Geometry: final body of the model. Coordinates: model frame, mm. Give positions to 0.01 mm unless a question says otherwise; leave off trailing zeros. Order: outer loops, then holes, each group sorted by start corner. A loop starts at its lowest first (then second) coordinate and runs counter-clockwise, first axis right, second up. Notation, with made-up numbers: (22.25, -8.5) - (66.25, -8.5) arc R33 cw to (66.25, 26.5) - close; hole circle Ø4 at (50.5, 66). An arc over 180 degrees is marked (long way). Use one line per item in the form item = value.
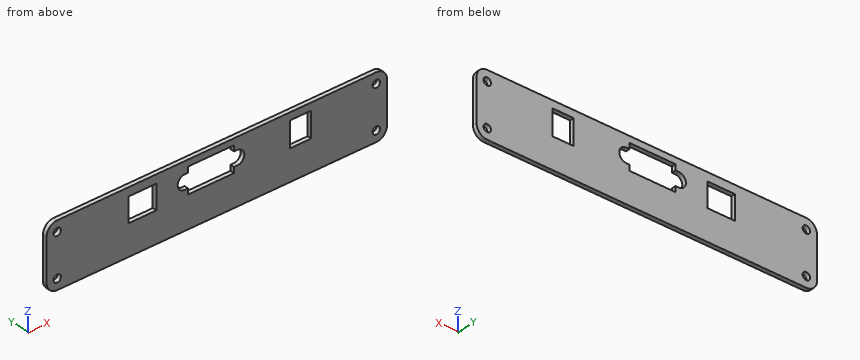
from build123d import *

# Parameters (mm, degrees)
SKETCH017_W          = 160
SKETCH017_H          = 30
PAD014_DEPTH         = 2
FILLET_R             = 5
SKETCH018_R          = 1.75
SKETCH018_W          = 13
SKETCH018_H          = 11.5
SKETCH018_W_2        = 10
SKETCH018_H_2        = 12
POCKET009_DEPTH      = 2.001
POCKET009_DEPTH_BACK = 0.001


with BuildPart() as part:
    # Sketch017 → Pad014 (new body)
    with BuildSketch(Plane.XZ):
        with Locations((0, 0.5)):
            Rectangle(SKETCH017_W, SKETCH017_H)
    extrude(amount=PAD014_DEPTH)

    # Fillet
    fillet_edges = [part.edges().sort_by_distance(p)[0] for p in [
        (80, -1, 15.5),
        (80, -1, -14.5),
        (-80, -1, 15.5),
        (-80, -1, -14.5),
    ]]
    fillet(fillet_edges, radius=FILLET_R)

    # Sketch018 (on Face5 of Pad014) → Pocket009 (cut, two sides)
    with BuildSketch(Plane(origin=(0, 0, 0), x_dir=(1, 0, 0), z_dir=(0, 1, 0))) as pocket009_sk:
        with Locations((-75, 9.5)):
            Circle(SKETCH018_R)
        with Locations((-75, -10.5)):
            Circle(SKETCH018_R)
        with Locations((75, 9.5)):
            Circle(SKETCH018_R)
        with Locations((75, -10.5)):
            Circle(SKETCH018_R)
        with BuildLine():
            Line((8.085, -12.5), (-13.515, -12.5))
            Line((-13.515, -12.5), (-13.515, -9.85))
            Line((-13.515, -9.85), (-15.015, -9.85))
            ThreePointArc((-15.015, -3.15), (-18.365, -6.5), (-15.015, -9.85))
            Line((-13.515, -3.15), (-15.015, -3.15))
            Line((-13.515, -0.5), (-13.515, -3.15))
            Line((8.085, -0.5), (-13.515, -0.5))
            Line((8.085, -3.15), (8.085, -0.5))
            Line((9.585, -3.15), (8.085, -3.15))
            ThreePointArc((9.585, -9.85), (12.935, -6.5), (9.585, -3.15))
            Line((8.085, -9.85), (9.585, -9.85))
            Line((8.085, -12.5), (8.085, -9.85))
        make_face()
        with Locations((-34.915, -5.75)):
            Rectangle(SKETCH018_W, SKETCH018_H)
        with Locations((39.385, -6)):
            Rectangle(SKETCH018_W_2, SKETCH018_H_2)
    extrude(amount=-POCKET009_DEPTH, mode=Mode.SUBTRACT)
    extrude(pocket009_sk.sketch, amount=POCKET009_DEPTH_BACK, mode=Mode.SUBTRACT)


solid = part.part
(1) Cut plane B-B on z = 6.5. Output: boundary loops of the cut face in (x, y) (3 decimals).
Computed values:
outline = (-80, -2) - (-41.415, -2) - (-41.415, 0) - (-80, 0) - close; (-28.415, -2) - (-18.365, -2) - (-18.365, 0) - (-28.415, 0) - close; (12.935, -2) - (34.385, -2) - (34.385, 0) - (12.935, 0) - close; (44.385, -2) - (80, -2) - (80, 0) - (44.385, 0) - close
(2) Cut plane A-A on x = -31. Output: boundary loops of the cut face in (y, z).
Computed values:
outline = (-2, -14.5) - (0, -14.5) - (0, 0) - (-2, 0) - close; (-2, 11.5) - (0, 11.5) - (0, 15.5) - (-2, 15.5) - close
(3) Ray query, line 1 along X through (y, z) = (-0.9, -9.5); line 2 along X through (y, z) = (-1.55, 10.5) (3 decimals); line 3 along Z through (x, y) = (-75, -1.1). Return the intervals inside material, ascending.
Computed values:
line_1 = -80 to -76.75, -73.25 to 73.25, 76.75 to 80
line_2 = -80 to -76.75, -73.25 to -41.415, -28.415 to -13.515, 8.085 to 34.385, 44.385 to 73.25, 76.75 to 80
line_3 = -14.5 to -11.25, -7.75 to 8.75, 12.25 to 15.5
(4) Cut plane C-C on y = -0.65. Give the number of separate pieces and of enclosed holes in the cut face, plus the area to 3 significant figures.
Computed values:
separate_pieces = 1
enclosed_holes = 7
area = 4,160 mm²
(5) Contact query for a flat-ended pin moving along its axis: pin 1 Ø4.5 at (x, z) = (75, -9.5) entering from -Y. Output: stop coordinate, or through.
Computed values:
pin_1 = -2
